Could you check a few things on this model? Use its own coordinates, in mm. A direction names the side the tool comes from. Coordinates: 2 decimals unless noted, no trailing zeros. Loops run counter-clockwise (first coordinate to the right, second up) from the corner with the lowest first, then second, coordinate; pieces in that order, holes last. Notation, with made-up numbers: (33.25, 61.25) -> (53.25, 61.25) arc R23 ccw to (53.25, 96.25) -> close; hole circle Ø10 at (-31, -20). An arc over 180 degrees is marked (long way). One line per question, with ' | ' between items.
from build123d import *

# Parameters (mm, degrees)
BOSS_EXTRUDE1_DEPTH   = 25.4
SKETCH2_R             = 2.75
CUT_EXTRUDE1_DEPTH    = 44.097043475
SKETCH3_R             = 4
CUT_EXTRUDE2_DEPTH    = 38.060560658
M2X0_4_TAPPED_HOLE1_D = 1.6


with BuildPart() as part:
    # Sketch1 → Boss-Extrude1 (new body)
    with BuildSketch(Plane.XY):
        Polygon((-11.1125, 0), (11.1125, 0), (11.1125, 23.8125), (12.7, 23.8125), (12.7, -1.5875), (-12.7, -1.5875), (-12.7, 23.8125), (-11.1125, 23.8125), align=None)
    extrude(amount=BOSS_EXTRUDE1_DEPTH)

    # Sketch2 → Cut-Extrude1 (cut, through all)
    with BuildSketch(Plane(origin=(12.7, 0, 0), x_dir=(0, 0, -1), z_dir=(1, 0, 0))):
        with Locations(Location((-12.7, 17.4625, 0), (0, 0, 90))):
            Circle(SKETCH2_R)
        with Locations(Location((-12.7, 6.35, 0), (0, 0, 90))):
            Circle(SKETCH2_R)
    extrude(amount=-CUT_EXTRUDE1_DEPTH, mode=Mode.SUBTRACT)

    # Sketch3 → Cut-Extrude2 (cut, through all)
    with BuildSketch(Plane(origin=(0, 0, 0), x_dir=(1, 0, 0), z_dir=(0, 1, 0))):
        with Locations(Location((0, -12.7, 0), (0, 0, 180))):
            Circle(SKETCH3_R)
    extrude(amount=-CUT_EXTRUDE2_DEPTH, mode=Mode.SUBTRACT)

    # M2x0.4 Tapped Hole1 (through all)
    with Locations(Plane(origin=(0, 0, 0), x_dir=(1, 0, 0), z_dir=(0, 1, 0))):
        with Locations((0, -6.458326036), (4.413529986, -8.286470014), (6.241673964, -12.7), (4.413529986, -17.113529986), (0, -18.941673964), (-4.413529986, -17.113529986), (-6.241673964, -12.7), (-4.413529986, -8.286470014)):
            Hole(M2X0_4_TAPPED_HOLE1_D / 2)


solid = part.part
1) I need wall thicknesses on line 1 along X through (y, z) = (13.25, 3.5); line 2 along Z through (x, y) = (12.2, 6.35); line 3 along Y through (x, z) = (6.5, 6). Which ranges of each line are inside material? Lowest first, please. Write a range as from..to.
Data:
line 1: -12.7..-11.11, 11.11..12.7 | line 2: 0..9.95, 15.45..25.4 | line 3: -1.59..0
2) If we section it at B-B on y = 6.35: Please give me the cut outline in (x, z).
Data:
outline: (-12.7, 0) -> (-11.11, 0) -> (-11.11, 9.95) -> (-12.7, 9.95) -> close; (-12.7, 15.45) -> (-11.11, 15.45) -> (-11.11, 25.4) -> (-12.7, 25.4) -> close; (11.11, 0) -> (12.7, 0) -> (12.7, 9.95) -> (11.11, 9.95) -> close; (11.11, 15.45) -> (12.7, 15.45) -> (12.7, 25.4) -> (11.11, 25.4) -> close
3) I'm going to push a flat-ended pin straight in: pin 1 Ø2 at (x, z) = (-6, 20.5) entering from +Y. Where does the tip first touch, or does it pass through?
Data:
pin 1: y = 0
4) If we section it at C-C on x = 2.5: Please give me the cut outline in (y, z).
Data:
outline: (-1.59, 0) -> (0, 0) -> (0, 9.58) -> (-1.59, 9.58) -> close; (-1.59, 15.82) -> (0, 15.82) -> (0, 25.4) -> (-1.59, 25.4) -> close
5) We'd pull the mould along Y, two halves only. Please class faces 3 (the face through (11.917, 4.323, 14.559)), 4 (the face through (-0.43, -0.805, 18.267)), 5 (the face through (-11.895, 4.323, 14.559)), 6 (the face through (3, -1.588, 9.7)): pulls with the +Y half, pulls with the -Y half, needs draft (parallel to the pull), parting line crosses it, or undercut.
Data:
face 3: undercut | face 4: needs draft | face 5: undercut | face 6: pulls with the -Y half
6) On a 3-axis mill with a long thin cutter (end or side, diameter ignored), from which of +Z, -Z, +X, -X, +Y, -Y can I reach the whole of each face in a straight line? I mean faces 1 (the face through (-11.112, 12, 13)), 2 (the face through (-4.309, -0.805, 7.493)). Say none if no direction works.
Data:
face 1: +Z, -Z, +Y | face 2: +Y, -Y
7) If we section it at A-A on y = 12.75: Please give me the cut outline in (x, z).
Data:
outline: (-12.7, 0) -> (-11.11, 0) -> (-11.11, 25.4) -> (-12.7, 25.4) -> close; (11.11, 0) -> (12.7, 0) -> (12.7, 25.4) -> (11.11, 25.4) -> close
8) If we section it at D-D on z = 3: Please give me the cut outline in (x, y), and give its area (3 significant figures).
Data:
outline: (-12.7, -1.59) -> (12.7, -1.59) -> (12.7, 23.81) -> (11.11, 23.81) -> (11.11, 0) -> (-11.11, 0) -> (-11.11, 23.81) -> (-12.7, 23.81) -> close | area: 116 mm²
